Input: part model. Units: mm. Frame: model coordinates. A direction names the side the tool comes from. Coordinates: 2 decimals unless noted, no trailing zeros. Order: outer loops, then holes, each group sorted by start corner. A loop starts at its lowest first (then second) coordinate and runs counter-clockwise, first axis right, second up. Notation, with made-up numbers: (-27.5, 43.25) -> (-0.5, 43.25) arc R20 cw to (-0.5, 57.25) -> close; hole circle Ø8 at (49.25, 25.25). An arc over 180 degrees is marked (long way). One line per question, with ' | ' between items.
```python
from build123d import *
from build123d.topology import SkipClean

# Parameters (mm, degrees)
SKETCH1_R           = 12.5
BOSS_EXTRUDE1_DEPTH = 100
SKETCH4_W           = 4
SKETCH4_H           = 27.5
BOSS_EXTRUDE3_DEPTH = 200
CIRPATTERN7_COUNT   = 4
SKETCH7_R           = 1.45
CUT_EXTRUDE2_DEPTH  = 27
CIRPATTERN9_COUNT   = 4
SKETCH10_R          = 12.5
BOSS_EXTRUDE4_DEPTH = 15


with BuildPart() as part:
    # Sketch1 → Boss-Extrude1 (new, symmetric)
    with BuildSketch(Plane.XY):
        Circle(SKETCH1_R)
    extrude(amount=BOSS_EXTRUDE1_DEPTH, both=True)

    # Sketch4 → Boss-Extrude3 (add)
    with BuildSketch(Plane.XY.offset(100)):
        with Locations((-7, 13.75)):
            Rectangle(SKETCH4_W, SKETCH4_H)
        with Locations((7, 13.75)):
            Rectangle(SKETCH4_W, SKETCH4_H)
    boss_extrude3 = extrude(amount=-BOSS_EXTRUDE3_DEPTH)

    # CirPattern7: Boss-Extrude3 ×4 about axis
    cirpattern7_axis = Axis((0, 0, 0), (0, 0, 1))
    for i in range(1, CIRPATTERN7_COUNT):
        add(boss_extrude3.rotate(cirpattern7_axis, i * 360 / CIRPATTERN7_COUNT))

    # Sketch7 → Cut-Extrude2 (cut)
    with BuildSketch(Plane.ZY.offset(9)):
        with Locations((-92.5, 20)):
            Circle(SKETCH7_R)
        with Locations((-52.5, 20)):
            Circle(SKETCH7_R)
        with Locations((-12.5, 20)):
            Circle(SKETCH7_R)
        with Locations((27.5, 20)):
            Circle(SKETCH7_R)
        with Locations((67.5, 20)):
            Circle(SKETCH7_R)
    cut_extrude2 = extrude(amount=-CUT_EXTRUDE2_DEPTH, mode=Mode.SUBTRACT)

    # CirPattern9: Cut-Extrude2 ×4 about axis
    cirpattern9_axis = Axis((0, 0, 100), (0, 0, 1))
    for i in range(1, CIRPATTERN9_COUNT):
        add(cut_extrude2.rotate(cirpattern9_axis, i * 360 / CIRPATTERN9_COUNT), mode=Mode.SUBTRACT)

    # Sketch10 → Boss-Extrude4 (add)
    with SkipClean():  # the faces are left unmerged after this step: merging them gives an invalid solid
        with BuildSketch(Plane(origin=(0, 0, -100), x_dir=(-1, 0, 0), z_dir=(0, 0, -1))):
            Circle(SKETCH10_R)
        extrude(amount=BOSS_EXTRUDE4_DEPTH)
    add(part.part.scale(1), mode=Mode.REPLACE)  # the faces are merged on a copy


solid = part.part
```
1. Pin query (flat end, axial travel): pin 1 Ø6 at (x, z) = (-15.5, -73) entering from -Y; pin 2 Ø1.7 at (y, z) = (20, 67.5) entering from -X; pin 3 Ø4 at (y, z) = (20, 27.5) entering from -X; pin 4 Ø4.5 at (x, z) = (-20, -52.5) entering from +Y. Return the tip coordinate at first contact, or that it passes through.
Recorded:
pin 1: stops at y = -9 | pin 2: passes through | pin 3: stops at x = -9 | pin 4: stops at y = 9
2. Mould query, pull axis X, two halves, no side actions, for faces 5 (the face through (5, -19, 1)), 6 (the face through (27.5, 7, 1)), 7 (the face through (-27.5, -7, 1)), 8 (the face through (19, 5, 1)). Classes: released by +X, released by -X, zero draft, split by the parting line, or undercut.
Recorded:
face 5: undercut | face 6: released by +X | face 7: released by -X | face 8: zero draft
3. Access query for faces 1 (the face through (-5, 19, 1)), 2 (the face through (-18, -9, 1)), 3 (the face through (-19, -5, 1)), 4 (the face through (9, 18, 1)). Directions: +Z, -Z, +X, -X, +Y, -Y. A direction counts if a zero-diameter tool reaches every point of the face in a straight line with its end or side. Return the directions, or none.
Recorded:
face 1: +Z, -Z, +Y | face 2: +Z, -Z, -X, -Y | face 3: +Z, -Z, -X | face 4: +Z, -Z, +X, +Y
4. Cut plane D-D, the plane x = 0. Return loops of the section in (y, z).
Recorded:
outline: (-12.5, -115) -> (12.5, -115) -> (12.5, 100) -> (-12.5, 100) -> close
5. Cut plane C-C, the plane z = 48.5. Return loops of the section in (x, y), and give its area (3 significant figures).
Recorded:
outline: (-27.5, -9) -> (-9, -9) -> (-9, -27.5) -> (-5, -27.5) -> (-5, -11.46) arc R12.5 ccw to (5, -11.46) -> (5, -27.5) -> (9, -27.5) -> (9, -9) -> (27.5, -9) -> (27.5, -5) -> (11.46, -5) arc R12.5 ccw to (11.46, 5) -> (27.5, 5) -> (27.5, 9) -> (9, 9) -> (9, 27.5) -> (5, 27.5) -> (5, 11.46) arc R12.5 ccw to (-5, 11.46) -> (-5, 27.5) -> (-9, 27.5) -> (-9, 9) -> (-27.5, 9) -> (-27.5, 5) -> (-11.46, 5) arc R12.5 ccw to (-11.46, -5) -> (-27.5, -5) -> close | area: 1,040 mm^2
6. Cut plane A-A, the plane y = 24.5. Return loops of the section in (x, z).
Recorded:
outline: (-9, -100) -> (-5, -100) -> (-5, 100) -> (-9, 100) -> close; (5, -100) -> (9, -100) -> (9, 100) -> (5, 100) -> close
7. Ray query, line 1 (Z direction, x = -7.2, y = -20); line 2 (X direction, y = -6.2, z = 67.5). Return the intervals inside material, ascending. Write a range as [from, to].
Recorded:
line 1: z = [-100, -93.95], [-91.05, -53.95], [-51.05, -13.95], [-11.05, 26.05], [28.95, 66.05], [68.95, 100] | line 2: x = [-27.5, -21.45], [-18.55, 18.55], [21.45, 27.5]
